For this review, take the finished solid that the model builds, in its own axes (mm). Face numbers are marked on the shaded views. A direction names the side the tool comes from. Round coordinates to 2 decimals unless told otherwise and drop trailing zeros. Write each loop counter-clockwise with the first axis right and the second up, starting at its lowest first coordinate (ties: lowest second). Pieces come first, ordered by that corner, then holes. Notation, with made-up numbers: M 87,-18.75 L 96,-18.75 A25 cw 96,-0.75 Z; hole C -6,-23.75 d6. An arc over 180 degrees is marked long. Answer in a Markdown table with one row per item.
```python
from build123d import *

# Parameters (mm, degrees)
BOSS_EXTRUDE1_DEPTH     = 24
FILLET1_R               = 4
CUT_EXTRUDE3_DEPTH      = 14
CUT_EXTRUDE3_DEPTH_BACK = 14
SKETCH5_R               = 2
CUT_EXTRUDE4_DEPTH      = 6
CUT_EXTRUDE4_DEPTH_BACK = 22
SKETCH7_W               = 14
SKETCH7_H               = 22.802557385
CUT_EXTRUDE5_DEPTH      = 1
CUT_EXTRUDE5_DEPTH_BACK = 27.278788925
FILLET2_R               = 2


with BuildPart() as part:
    # Sketch1 → Boss-Extrude1 (new body)
    with BuildSketch(Plane(origin=(0, 0, 0), x_dir=(1, 0, 0), z_dir=(0, 1, 0))):
        with BuildLine():
            Line((18, -8), (10.246950766, -8))
            ThreePointArc((10.246950766, -8), (-13, 0), (10.246950766, 8))
            Line((10.246950766, 8), (18, 8))
            Line((18, 8), (18, -8))
        make_face()
        with BuildLine():
            Line((17, -7), (9.746794345, -7))
            ThreePointArc((9.746794345, -7), (-12, 0), (9.746794345, 7))
            Line((9.746794345, 7), (17, 7))
            Line((17, 7), (17, -7))
        make_face(mode=Mode.SUBTRACT)
    extrude(amount=BOSS_EXTRUDE1_DEPTH)

    # Fillet1
    fillet1_edges = [part.edges().sort_by_distance(p)[0] for p in [
        (9.746794345, 12, -7),
        (9.746794345, 12, 7),
        (10.246950766, 12, 8),
        (10.246950766, 12, -8),
    ]]
    fillet(fillet1_edges, radius=FILLET1_R)

    # Sketch4 → Cut-Extrude3 (cut, two sides)
    with BuildSketch(Plane.XY) as cut_extrude3_sk:
        Polygon((-13, 0), (-8.278788925, 0), (9.208278207, 24), (-13, 24), align=None)
    extrude(amount=CUT_EXTRUDE3_DEPTH, mode=Mode.SUBTRACT)
    extrude(cut_extrude3_sk.sketch, amount=-CUT_EXTRUDE3_DEPTH_BACK, mode=Mode.SUBTRACT)

    # Sketch5 → Cut-Extrude4 (cut, two sides)
    with BuildSketch(Plane.XY.offset(8)) as cut_extrude4_sk:
        with Locations((15, 17.5)):
            Circle(SKETCH5_R)
    extrude(amount=CUT_EXTRUDE4_DEPTH, mode=Mode.SUBTRACT)
    extrude(cut_extrude4_sk.sketch, amount=-CUT_EXTRUDE4_DEPTH_BACK, mode=Mode.SUBTRACT)

    # Sketch7 → Cut-Extrude5 (cut, two sides)
    with BuildSketch(Plane(origin=(18, 0, 0), x_dir=(0, 0, -1), z_dir=(1, 0, 0))) as cut_extrude5_sk:
        with Locations((0, 14.401278693)):
            Rectangle(SKETCH7_W, SKETCH7_H)
    extrude(amount=CUT_EXTRUDE5_DEPTH, mode=Mode.SUBTRACT)
    extrude(cut_extrude5_sk.sketch, amount=-CUT_EXTRUDE5_DEPTH_BACK, mode=Mode.SUBTRACT)

    # Fillet2
    fillet2_edges = [part.edges().sort_by_distance(p)[0] for p in [
        (17.5, 3, -7),
        (17.5, 3, 7),
    ]]
    fillet(fillet2_edges, radius=FILLET2_R)


solid = part.part
```
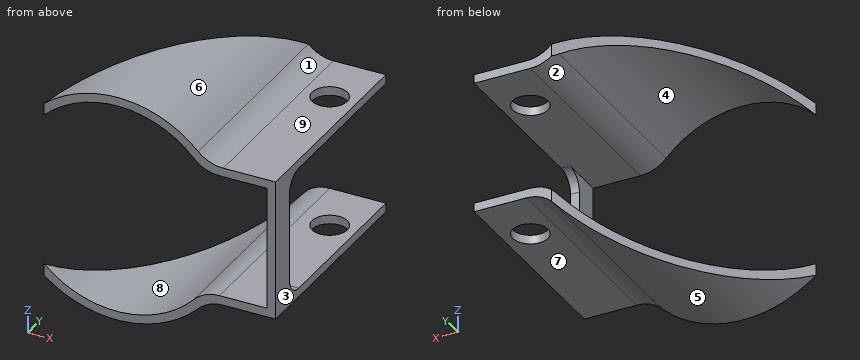
Q1. Take a section at A-A (x = 15). State the section outline as (y, z) points.
Found:
| item | result |
|---|---|
| outline | M 0,-8 L 15.5,-8 L 15.5,-7 L 0,-7 Z; M 0,7 L 15.5,7 L 15.5,8 L 0,8 Z; M 19.5,-8 L 24,-8 L 24,-7 L 19.5,-7 Z; M 19.5,7 L 24,7 L 24,8 L 19.5,8 Z |
Q2. For probe 1 along Z at (x, y) = (12.25, 10.75); probe 2 along Y at (x, z) = (15, 7.5); probe 3 along Z at (x, y) = (0.5, 9.75), list the stretches that pass through material, from the lowest coordinate up.
Found:
| item | result |
|---|---|
| probe 1 | -8 to -7, 7 to 8 |
| probe 2 | 0 to 15.5, 19.5 to 24 |
| probe 3 | -12.99 to -11.99, 11.99 to 12.99 |
Q3. Take a section at B-B (z = -11). State the section outline as (x, y) points.
Found:
| item | result |
|---|---|
| outline | M -6.93,0 L -4.8,0 L -4.8,4.78 L -6.93,1.85 Z; M 4.8,0 L 6.93,0 L 6.93,20.87 L 4.8,17.94 Z |
Q4. Machinability: for the marked faces 5, 6, 7, 8 and 9, which of the approach directions +Z, -Z, +X, -X, +Y, -Y give a long, thin tool a straight path to every point of the face, cutting with its end or side? Answer none if there is none.
Found:
| item | result |
|---|---|
| face 5 | -Z, +Y, -Y |
| face 6 | +Z, +Y, -Y |
| face 7 | -Z, +X, +Y, -Y |
| face 8 | +Y, -Y |
| face 9 | +Z, +X, +Y, -Y |
Q5. Insertion check: P1, Ø6, axis at x = -2.5, y = 16.5, coming from the -Z side; P2, Ø1.8, axis at x = 16.5, y = 7.5, coming from the -Z side; P3, Ø3, axis at x = 11.5, z = 8.5, coming from the +Y side; P4, Ø1, axis at x = 9.5, y = 4.5, coming from the +Z side. Each pin has a flat end and moves straight along its axis. Give the tip position at first contact, or say it passes through.
Found:
| item | result |
|---|---|
| P1 | through |
| P2 | z = -8 |
| P3 | y = 24 |
| P4 | z = 9.38 |
Q6. Take a section at C-C (x = 7.75). State the section outline as (y, z) points.
Found:
| item | result |
|---|---|
| outline | M 0,-10.44 L 22,-10.44 L 22,-9.16 L 0,-9.16 Z; M 0,9.16 L 22,9.16 L 22,10.44 L 0,10.44 Z |
Q7. Take a section at D-D (y = 14.25). State the section outline as (x, z) points, then the cut area to 3 significant figures.
Found:
| item | result |
|---|---|
| outline | M 2.1,-12.83 A13 ccw 9.21,-9.18 A4 cw 12.04,-8 L 18,-8 L 18,-7 L 11.62,-7 A4 ccw 8.71,-8.25 A12 cw 2.1,-11.81 Z; M 2.1,11.81 A12 cw 8.71,8.25 A4 ccw 11.62,7 L 18,7 L 18,8 L 12.04,8 A4 cw 9.21,9.18 A13 ccw 2.1,12.83 Z |
| area | 34.9 mm² |
Q8. Mouldability with a two-part tool opening along Z and no side actions: class the marked faces 1, 2, 3 and 4 as +Z half, -Z half, draft (parallel to the pull), parting line (faces both ways), or undercut.
Found:
| item | result |
|---|---|
| face 1 | +Z half |
| face 2 | undercut |
| face 3 | draft |
| face 4 | undercut |
